The listing builds one solid part. Answer for the finished solid, in the listing's coordinates (mm). A direction names the side the tool comes from. Coordinates: 2 decimals unless noted, no trailing zeros. Write each loop counter-clockwise with the first axis right and the second up, starting at its lowest first coordinate (ties: lowest second). Pieces come first, ordered by that corner, then holes.
(1) The part is cut by section D-D on x = -24. Determine the outline of the cut face in (y, z).
(2) Straight lines are drawn through the part: line 1 (X direction, y = -25.25, z = -15.2); line 2 (X direction, y = -19.45, z = -15.2); line 3 (X direction, y = -15.5, z = 1). For each, find the intervals that lie inside material, in ascending order.
(3) Which of the six approach directions +Z, -Z, +X, -X, +Y, -Y give full straight-line access (tool end or side, diameter ignored) to faces 1 (the flat face through (15, -8, 0)), 2 (the flat face through (12, -21.2, -13)), 3 (the cylindrical face through (14.02, -5.68, 13.07))?
(4) The part is cut by section A-A on y = -26. Determine the outline of the cut face in (x, z), plus the area to 3 significant figures.
(5) Given P1, Ø3, axis at x = -14.5, y = -13.5, coming from the +Z side; P2, Ø10, axis at x = -15, z = -15.2, coming from the +Y side; P3, Ø5, axis at y = -4, z = 12.5, coming from the +X side; P4, Ø9.5, axis at x = 14.8, z = -15.2, coming from the -Y side, each flat-ended and moving along its own axis, determine where each tip first touches the part or whether it passes through.
(6) For a pull along Z with two mould halves and no side action, classify faces 4 (the flat face through (18, -17, 18)), 5 (the cylindrical face through (3, -3.2, 14.9)), 6 (the flat face through (29.8, -28, -8)) as +Z half, -Z half, draft (parallel to the pull), parting line (faces both ways), or undercut.
(7) The part is cut by section C-C on x = -15. Determine the outline of the cut face in (y, z), plus the area to 3 significant figures.
(8) The part is cut by section B-B on z = -15.2. Determine the outline of the cut face in (x, y), plus the area to 3 significant figures.
from build123d import *

# Parameters (mm, degrees)
BOSS_EXTRUDE1_DEPTH = 29.8
BOSS_EXTRUDE2_DEPTH = 30
SKETCH2_R           = 3.2
CUT_EXTRUDE1_DEPTH  = 62.943845538
CUT_EXTRUDE2_START  = -21.2
SKETCH2_3_R         = 6
SKETCH2_3_R_2       = 3.2
CUT_EXTRUDE2_DEPTH  = 41.743845538
CUT_EXTRUDE3_START  = 6
CUT_EXTRUDE3_DEPTH  = 56.943845538


with BuildPart() as part:
    # Sketch1 → Boss-Extrude1 (new body)
    with BuildSketch(Plane.YZ):
        with BuildLine():
            Line((-15.2, 0), (0, 0))
            Line((0, 0), (0, 11.8))
            ThreePointArc((0, 11.8), (-3.2, 15), (0, 18.2))
            Line((0, 18.2), (0, 30))
            Line((0, 30), (-21.2, 30))
            Line((-21.2, 30), (-45, 6.2))
            Line((-45, 6.2), (-45, -6.4))
            Line((-45, -6.4), (-21.2, -30.2))
            Line((-21.2, -30.2), (-15.2, -30.2))
            Line((-15.2, -30.2), (-15.2, 0))
        make_face()
    extrude(amount=BOSS_EXTRUDE1_DEPTH)

    # Sketch1<3> → Boss-Extrude2 (add)
    with BuildSketch(Plane.YZ):
        Polygon((-15.2, -30.2), (-15.2, -0.2), (-45, -0.2), (-45, -6.4), (-21.2, -30.2), align=None)
    extrude(amount=-BOSS_EXTRUDE2_DEPTH)

    # Sketch2 → Cut-Extrude1 (cut, through all)
    with BuildSketch(Plane(origin=(0, 0, 0), x_dir=(-1, 0, 0), z_dir=(0, 1, 0))):
        Polygon((-29.8, 18.2), (-17.8, 18.2), (-6, 30), (-29.8, 30), align=None)
        Polygon((-29.8, 11.8), (-24.2, 11.8), (-17.8, 18.2), (-29.8, 18.2), align=None)
        Polygon((-29.8, 11.8), (-29.8, 6.2), (-24.2, 11.8), align=None)
        with Locations(Location((-14.8, -15.2, 0), (0, 0, 90))):
            Circle(SKETCH2_R)
        with Locations(Location((15, -15.2, 0), (0, 0, 90))):
            Circle(SKETCH2_R)
    extrude(amount=-CUT_EXTRUDE1_DEPTH, mode=Mode.SUBTRACT)

    # Sketch2<3> → Cut-Extrude2 (cut, through all)
    # profile 1 of 2: a face of its own
    with BuildSketch(Plane(origin=(0, 0, 0), x_dir=(-1, 0, 0), z_dir=(0, 1, 0)).offset(CUT_EXTRUDE2_START)):
        with Locations(Location((-14.8, -15.2, 0), (0, 0, 90))):
            Circle(SKETCH2_3_R)
        with Locations(Location((-14.8, -15.2, 0), (0, 0, 90))):
            Circle(SKETCH2_3_R_2, mode=Mode.SUBTRACT)
    # profile 2 of 2: a face of its own
    with BuildSketch(Plane(origin=(0, 0, 0), x_dir=(-1, 0, 0), z_dir=(0, 1, 0)).offset(CUT_EXTRUDE2_START)):
        with Locations(Location((15, -15.2, 0), (0, 0, 90))):
            Circle(SKETCH2_3_R)
        with Locations(Location((15, -15.2, 0), (0, 0, 90))):
            Circle(SKETCH2_3_R_2, mode=Mode.SUBTRACT)
    extrude(amount=-CUT_EXTRUDE2_DEPTH, mode=Mode.SUBTRACT)

    # Sketch1<4> → Cut-Extrude3 (cut, through all)
    with BuildSketch(Plane.YZ.offset(CUT_EXTRUDE3_START)):
        with BuildLine():
            ThreePointArc((0, 21), (-6, 15), (0, 9))
            Line((0, 9), (0, 11.8))
            ThreePointArc((0, 11.8), (-3.2, 15), (0, 18.2))
            Line((0, 18.2), (0, 21))
        make_face()
        with BuildLine():
            Line((0, 11.8), (0, 9))
            ThreePointArc((0, 9), (4.242640687, 10.757359313), (6, 15))
            ThreePointArc((6, 15), (4.242640687, 19.242640687), (0, 21))
            Line((0, 21), (0, 18.2))
            ThreePointArc((0, 18.2), (2.2627417, 17.2627417), (3.2, 15))
            ThreePointArc((3.2, 15), (2.2627417, 12.7372583), (0, 11.8))
        make_face()
    extrude(amount=CUT_EXTRUDE3_DEPTH, mode=Mode.SUBTRACT)


solid = part.part
Model answer:
1. outline: (-45, -6.4) - (-21.2, -30.2) - (-15.2, -30.2) - (-15.2, -0.2) - (-45, -0.2) - close
2. line 1: x = -30 to -21, -9 to 8.8, 20.8 to 29.8
2. line 2: x = -30 to -18.2, -11.8 to 11.6, 18 to 29.8
2. line 3: x = 0 to 29.8
3. face 1: -Z, +X, -X, +Y
3. face 2: -Y
3. face 3: +X, +Y
4. outline: (-30, -25.4) - (29.8, -25.4) - (29.8, 6.2) - (10.8, 25.2) - (0, 25.2) - (0, -0.2) - (-30, -0.2) - close; hole circle Ø12 at (-15, -15.2); hole circle Ø12 at (14.8, -15.2)
4. area: 1,860 mm2
5. P1: passes through
5. P2: stops at y = -15.2
5. P3: stops at x = 26
5. P4: stops at y = -21.2
6. face 4: +Z half
6. face 5: undercut
6. face 6: draft
7. outline: (-45, -6.4) - (-42.2, -9.2) - (-21.2, -9.2) - (-21.2, -12) - (-15.2, -12) - (-15.2, -0.2) - (-45, -0.2) - close; (-30.2, -21.2) - (-21.2, -30.2) - (-15.2, -30.2) - (-15.2, -18.4) - (-21.2, -18.4) - (-21.2, -21.2) - close
7. area: 392 mm2
8. outline: (-30, -36.2) - (-21, -36.2) - (-21, -21.2) - (-18.2, -21.2) - (-18.2, -15.2) - (-30, -15.2) - close; (-11.8, -21.2) - (-9, -21.2) - (-9, -36.2) - (8.8, -36.2) - (8.8, -21.2) - (11.6, -21.2) - (11.6, -15.2) - (-11.8, -15.2) - close; (18, -21.2) - (20.8, -21.2) - (20.8, -36.2) - (29.8, -36.2) - (29.8, -15.2) - (18, -15.2) - close
8. area: 819 mm2
